```python
from build123d import *

# Parameters (mm, degrees)
F0_W      = 184.15
F0_H      = 50.8
F1_DEPTH  = 3.175
F3_D      = 3.2
F4_W      = 184.15
F4_H      = 3.175
F5_DEPTH  = 76.2
F7_D      = 3.3
F8_W      = 3.175
F8_H      = 47.625
F9_DEPTH  = 76.2
F10_W     = 19.05
F10_H     = 34.925
F11_DEPTH = 3.175
F12_W     = 3.175
F12_H     = 47.625
F13_DEPTH = 76.2
F14_W     = 13.2291666667
F14_H     = 31.75
F14_W_2   = 11.6416666667
F15_DEPTH = 3.175
F16_W     = 6.35
F16_H     = 6.35
F17_DEPTH = 6.35
F19_D     = 2.4
F19_DEPTH = 12.7
F19_TIP   = 0.7210327428
F20_W     = 121.4
F20_H     = 34.925
F21_DEPTH = 25.4
F22_W     = 60.2
F22_H     = 32.26
F23_DEPTH = 25.4
F25_DEPTH = 50.801
F27_D     = 2.4
F27_DEPTH = 12.7
F27_TIP   = 0.7210327428


with BuildPart() as f1:
    # F0 (on Top) → F1 (new body)
    with BuildSketch(Plane.XY):
        with Locations((-3.8965528874, 0)):
            Rectangle(F0_W, F0_H)
    extrude(amount=F1_DEPTH)

    # F3 (through all)
    with Locations(Plane.XY.offset(3.175)):
        with Locations((-78.8965528874, 9.525), (-78.8965528874, -15.475), (71.1034471126, -15.475), (71.1034471126, 9.525)):
            Hole(F3_D / 2)

    # F4 (on face) → F5 (join)
    with BuildSketch(Plane.XY.offset(3.175)):
        with Locations((-3.8965528874, 23.8125)):
            Rectangle(F4_W, F4_H)
    extrude(amount=F5_DEPTH)

    # F7 (through all)
    with Locations(Plane.XZ.offset(-22.225)):
        with Locations((-70.5715528874, 66.675), (11.9784471126, 66.675), (10.7084471126, 18.415), (-64.2215528874, 18.415)):
            Hole(F7_D / 2)

    # F8 (on face) → F9 (join)
    with BuildSketch(Plane.XY.offset(3.175)):
        with Locations((-94.3840528874, -1.5875)):
            Rectangle(F8_W, F8_H)
    extrude(amount=F9_DEPTH)

    # F10 (on face) → F11 (cut, through all)
    with BuildSketch(Plane(origin=(-95.9715528874, 0, 0), x_dir=(0, -1, 0), z_dir=(-1, 0, 0))):
        with Locations((12.7, 58.7375)):
            Rectangle(F10_W, F10_H)
        with Locations((12.7, 20.6375)):
            Rectangle(F10_W, F10_H)
    extrude(amount=-F11_DEPTH, mode=Mode.SUBTRACT)

    # F12 (on face) → F13 (join)
    with BuildSketch(Plane.XY.offset(3.175)):
        with Locations((86.5909471126, -1.5875)):
            Rectangle(F12_W, F12_H)
    extrude(amount=F13_DEPTH)

    # F14 (on face) → F15 (cut, through all)
    with BuildSketch(Plane.YZ.offset(88.1784471126)):
        with Locations((-15.6104166667, 19.05)):
            Rectangle(F14_W, F14_H)
        with Locations((0, 19.05)):
            Rectangle(F14_W_2, F14_H)
        with Locations((15.6104166667, 19.05)):
            Rectangle(F14_W, F14_H)
    extrude(amount=-F15_DEPTH, mode=Mode.SUBTRACT)

    # F16 (on face) → F17 (join)
    with BuildSketch(Plane.XZ.offset(-22.225)):
        with Locations((-89.6215528874, 76.2)):
            Rectangle(F16_W, F16_H)
        with Locations((81.8284471126, 76.2)):
            Rectangle(F16_W, F16_H)
    extrude(amount=F17_DEPTH)

    # F19
    with Locations(Plane.XY.offset(79.375)):
        with Locations((-89.6215528874, 19.05), (81.8284471126, 19.05)):
            Hole(F19_D / 2, depth=F19_DEPTH)
            with Locations((0, 0, -(F19_DEPTH + F19_TIP / 2))):  # 118° drill point
                Cone(0, F19_D / 2, F19_TIP, mode=Mode.SUBTRACT)

    # F20 (on face) → F21 (cut)
    with BuildSketch(Plane.XY.offset(3.175)):
        with Locations((-3.8965528874, -1.5875)):
            Rectangle(F20_W, F20_H)
    extrude(amount=-F21_DEPTH, mode=Mode.SUBTRACT)

    # F22 (on face) → F23 (cut)
    with BuildSketch(Plane.XZ.offset(-22.225)):
        with Locations((-26.1215528874, 42.545)):
            Rectangle(F22_W, F22_H)
    extrude(amount=-F23_DEPTH, mode=Mode.SUBTRACT)

    # F24 (on face) → F25 (cut, through all)
    with BuildSketch(Plane.XZ.offset(25.4)):
        Polygon((-92.7965528874, 79.375), (-95.9715528874, 79.375), (-95.9715528874, 0), (85.0034471126, 0), (85.0034471126, 3.175), (-92.7965528874, 3.175), align=None)
    extrude(amount=-F25_DEPTH, mode=Mode.SUBTRACT)

    # F27
    with Locations(Plane.XZ.offset(-22.225)):
        with Locations((-89.6215528874, 6.35), (81.8284471126, 6.35)):
            Hole(F27_D / 2, depth=F27_DEPTH)
            with Locations((0, 0, -(F27_DEPTH + F27_TIP / 2))):  # 118° drill point
                Cone(0, F27_D / 2, F27_TIP, mode=Mode.SUBTRACT)


solid = f1.part
```
The model under review builds one solid part; all positions refer to its coordinate system, in mm. A direction names the side the tool comes from. Round coordinates to 2 decimals unless told otherwise and drop trailing zeros. Loops run counter-clockwise (first coordinate to the right, second up) from the corner with the lowest first, then second, coordinate; pieces in that order, holes last. Notation, with made-up numbers: (44.5, 75.5) - (62.5, 75.5) arc R3 ccw to (62.5, 80.5) - close; hole circle Ø10 at (-16, -7). An arc over 180 degrees is marked (long way). Write each question's results on one line, items separated by ' | '. Start each with the question number.
Q1. Insertion check: P1, Ø2, axis at x = 7, z = 20.5, coming from the -Y side (3 decimals); P2, Ø1, axis at x = -2.5, y = 24.5, coming from the -Z side (3 decimals); P3, Ø5, axis at x = -90, y = 18.5, coming from the -Z side (3 decimals). Each pin has a flat end and moves straight along its axis. Give the tip position at first contact, or say it passes through.
Q2. Take a section at D-D on z = 42.5. Give the boundary of the cut face in (x, y) (3 decimals).
Q3. Wall thickness on line 1 along X through (y, z) = (19, 75); line 2 along Y through (x, z) = (42, 29.5) (3 decimals); line 3 along X through (y, z) = (11, 41.5): over which ranges is each line inside the solid? List them lowest first. Write a range as [from, to].
Q4. Take a section at A-A on x = -21.5. Give the boundary of the cut face in (y, z) (3 decimals).
Q5. Take a section at B-B on z = 23. Give the boundary of the cut face in (x, y) (3 decimals), plus the area to 3 significant figures.
Q6. Draft analysis for pull direction Y (two halves, no side actions). For faces 6 (the flat face through (-27, 24, 26.415)), 7 (the flat face through (87, -25.4, 39)), 8 (the flat face through (87, -22.225, 19)), state which applies: pulls with the +Y half, pulls with the -Y half, needs draft (parallel to the pull), parting line crosses it, or undercut.
Q7. Take a section at C-C on y = -11. Give the boundary of the cut face in (x, z) (3 decimals), plus the area to 3 significant figures.
Q8. Tool access review of faces 1 (the flat face through (-90, 15.875, 76)), 2 (the flat face through (81.8, 17.7, 73.025)), 3 (the flat face through (-3, 24, 3.175)), 4 (the flat face through (87, -5.821, 19)), 5 (the flat face through (-27, 24, 58.675)): name each direction out of +Z, -Z, +X, -X, +Y, -Y from which nothing blocks a thin tool from reaching the whole face with its end or side.
Data:
1) P1: stops at y = 22.225 | P2: stops at z = 3.175 | P3: stops at z = 73.025
2) outline: (-92.797, 22.225) - (-56.222, 22.225) - (-56.222, 25.4) - (-92.797, 25.4) - close; (3.978, 22.225) - (85.003, 22.225) - (85.003, -25.4) - (88.178, -25.4) - (88.178, 25.4) - (3.978, 25.4) - close
3) line 1: x = [-92.8, -90.82], [-88.42, -86.45], [78.65, 80.63], [83.03, 88.18] | line 2: y = [22.225, 25.4] | line 3: x = [85, 88.18]
4) outline: (22.225, 3.175) - (25.4, 3.175) - (25.4, 26.415) - (22.225, 26.415) - close; (22.225, 58.675) - (25.4, 58.675) - (25.4, 79.375) - (22.225, 79.375) - close
5) outline: (-92.797, 22.225) - (88.178, 22.225) - (88.178, 25.4) - (-92.797, 25.4) - close; (85.003, -25.4) - (88.178, -25.4) - (88.178, -22.225) - (85.003, -22.225) - close; (85.003, -8.996) - (88.178, -8.996) - (88.178, -5.821) - (85.003, -5.821) - close; (85.003, 5.821) - (88.178, 5.821) - (88.178, 8.996) - (85.003, 8.996) - close | area: 605 mm²
6) face 6: needs draft | face 7: pulls with the -Y half | face 8: undercut
7) outline: (85.003, 0) - (88.178, 0) - (88.178, 3.175) - (85.003, 3.175) - close; (85.003, 34.925) - (88.178, 34.925) - (88.178, 79.375) - (85.003, 79.375) - close | area: 151 mm²
8) face 1: +Z, -Z, -X, -Y | face 2: -Z, -X, -Y | face 3: -Z, -X, +Y, -Y | face 4: +X, -X | face 5: +Y, -Y
